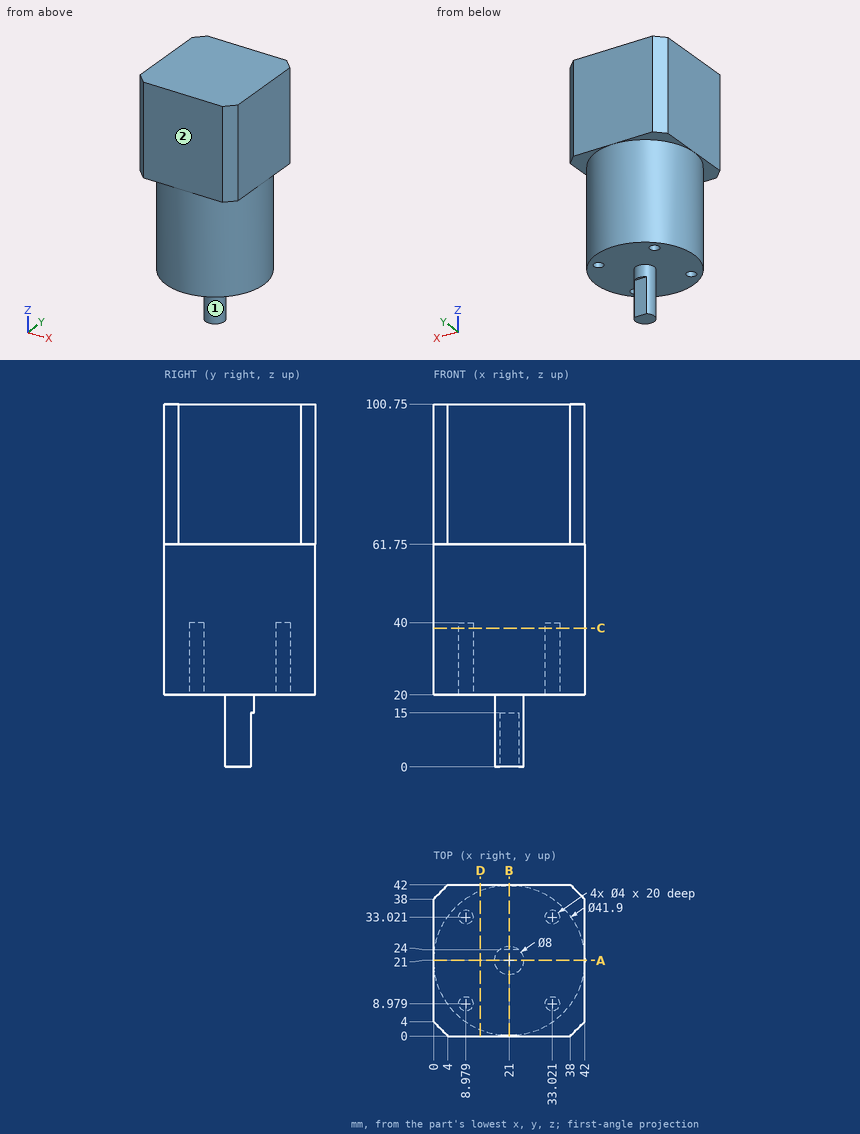
Source: three-view drawing plus pictorial views. Frame: mm from the lowest corner of the part. A direction names the side the tool comes from. Coordinates: 2 decimals unless noted, no trailing zeros. Write each loop counter-clockwise with the first axis right and the second up, starting at its lowest first coordinate (ties: lowest second). Pieces come first, ordered by that corner, then holes. Notation, with made-up numbers: (71, 44.5) -> (95, 44.5) arc R26 cw to (95, 61.5) -> close; hole circle Ø2 at (16.25, -31.5). An arc over 180 degrees is marked (long way). Answer as a JSON object with one key per item and string values.
1. Section C-C on z = 38.5. Return the cut outline in (x, y).
Result set:
{"outline": "circle Ø41.9 at (21, 21); hole circle Ø4 at (8.98, 8.98); hole circle Ø4 at (8.98, 33.02); hole circle Ø4 at (33.02, 8.98); hole circle Ø4 at (33.02, 33.02)"}
2. Section B-B on x = 21. Return the cut outline in (y, z).
Result set:
{"outline": "(0, 61.75) -> (0.05, 61.75) -> (0.05, 20) -> (17, 20) -> (17, 0) -> (24, 0) -> (24, 15) -> (25, 15) -> (25, 20) -> (41.95, 20) -> (41.95, 61.75) -> (42, 61.75) -> (42, 100.75) -> (0, 100.75) -> close"}
3. Material intervals for line 1 (X direction, y = 10.5, z = 27); line 2 (Z direction, x = 20.5, y = 25); line 3 (Z direction, x = 20.5, y = 24.5), sorted ascending. Write a range as from..to.
Result set:
{"line 1": "x = 2.87..7.68, 10.28..31.72, 34.32..39.13", "line 2": "z = 20..100.75", "line 3": "z = 15..100.75"}
4. Access query for the marked faces 1 and 2. Directions: +Z, -Z, +X, -X, +Y, -Y. A direction counts if a zero-diameter tool reaches every point of the face in a straight line with its end or side. Return the directions, or none.
Result set:
{"face 1": "-Z", "face 2": "+Z, -Z, +X, -X, -Y"}
5. Section D-D on x = 13. Return the cut outline in (y, z).
Result set:
{"outline": "(0, 61.75) -> (1.64, 61.75) -> (1.64, 20) -> (40.36, 20) -> (40.36, 61.75) -> (42, 61.75) -> (42, 100.75) -> (0, 100.75) -> close"}
6. Section A-A on y = 21. Return the cut outline in (x, z).
Result set:
{"outline": "(0, 61.75) -> (0.05, 61.75) -> (0.05, 20) -> (17, 20) -> (17, 0) -> (25, 0) -> (25, 20) -> (41.95, 20) -> (41.95, 61.75) -> (42, 61.75) -> (42, 100.75) -> (0, 100.75) -> close"}
7. First-contact query: P1, Ø1.2, axis at x = 33.5, y = 9, coming from the -Z side; P2, Ø5, axis at x = 10.5, y = 32.5, coming from the -Z side; P3, Ø6, axis at x = 20.5, z = 4, coming from the +Y side. Flat tips, straight axial feed; report the tip coordinate or a pass-through.
Result set:
{"P1": "stops at z = 40", "P2": "stops at z = 20", "P3": "stops at y = 24"}
